The model under review builds one solid part; all positions refer to its coordinate system, in mm. A direction names the side the tool comes from. Round coordinates to 2 decimals unless told otherwise and drop trailing zeros. Loops run counter-clockwise (first coordinate to the right, second up) from the corner with the lowest first, then second, coordinate; pieces in that order, holes last. Notation, with made-up numbers: (31, -23.5) -> (46, -23.5) arc R12 cw to (46, -19.5) -> close; hole circle Ø9 at (56.25, 60.25). An arc over 180 degrees is marked (long way). Use a Markdown table: item, result. Add a question column.
1) Mouldability with a two-part tool opening along Y and no side actions: class faces 1 (the cylindrical face through (31.1, -49, 3.1)), 2 (the flat face through (33.02, -1, 3)), 3 (the cylindrical face through (-31.1, 49, 3.1)), 4 (the cylindrical face through (-18.945, 34.933, 3.131)) as released by +Y, released by -Y, zero draft, split by the parting line, or undercut.
2) Wall thickness on probe 1 along X at (y, z) = (36, 3); probe 2 along Y at (x, z) = (-25, 5); probe 3 along Y at (x, z) = (0, 32): over which ranges is each line inside the solid? List them lowest first.
3) Consider section B-B on x = 0. Give the boundary of the cut face in (y, z).
4) Consider section C-C on y = 23. Give the boundary of the cut face in (x, z), plus the area to 3 significant figures.
5) Consider section D-D on z = 19. Give the boundary of the cut face in (x, y).
6) Insertion check: pin 1 (3 mm diameter, centred on x = -20.5, z = 9, fed in from +Y); pin 2 (1.5 mm diameter, centred on y = -24.5, z = 26, fed in from +X); pin 3 (5 mm diameter, centred on x = 26.5, z = 51, fed in from -Y). Each pin has a flat end and moves straight along its axis. Give the tip position at first contact, or say it passes through.
7) For faces 5 (the flat face through (0, 37, 6.35)), 6 (the cylindrical face through (15.237, -29.294, 33.273)), 7 (the flat face through (0, -36, 6.35)), 8 (the cylindrical face through (2.198, 31.543, 33.875)), list the 3-axis set-ups (+Z, -Z, +X, -X, +Y, -Y) from which the entire face can be reached by the end or side of a thin tool; tool diameter is ignored.
8) Consider section A-A on y = 36.83. Give the boundary of the cut face in (x, z).
from build123d import *

# Parameters (mm, degrees)
F0_R     = 4.953
F0_R_2   = 30.48
F1_DEPTH = 6.35
F2_R     = 33.02
F2_R_2   = 30.48
F3_DEPTH = 54.61
F5_D     = 9.525
F5_DEPTH = 50.801


with BuildPart() as f1:
    # F0 (on Top) → F1 (new body)
    with BuildSketch(Plane.XY):
        with BuildLine():
            ThreePointArc((33.02, 44.45), (31.1601280605, 48.9401280605), (26.67, 50.8))
            Line((26.67, 50.8), (-26.67, 50.8))
            ThreePointArc((-26.67, 50.8), (-31.1601280605, 48.9401280605), (-33.02, 44.45))
            Line((-33.02, 44.45), (-33.02, -44.45))
            ThreePointArc((-33.02, -44.45), (-31.1601280605, -48.9401280605), (-26.67, -50.8))
            Line((-26.67, -50.8), (26.67, -50.8))
            ThreePointArc((26.67, -50.8), (31.1601280605, -48.9401280605), (33.02, -44.45))
            Line((33.02, -44.45), (33.02, 44.45))
        make_face()
        with Locations((-25.4, -36.83)):
            Circle(F0_R, mode=Mode.SUBTRACT)
        with Locations((25.4, -36.83)):
            Circle(F0_R, mode=Mode.SUBTRACT)
        Circle(F0_R_2, mode=Mode.SUBTRACT)
        with Locations((-23.5207291554, 36.83)):
            Circle(F0_R, mode=Mode.SUBTRACT)
        with Locations((25.4, 36.83)):
            Circle(F0_R, mode=Mode.SUBTRACT)
    extrude(amount=F1_DEPTH)

    # F2 (on face) → F3 (join)
    with BuildSketch(Plane.XY.offset(6.35)):
        Circle(F2_R)
        Circle(F2_R_2, mode=Mode.SUBTRACT)
    extrude(amount=F3_DEPTH)

    # F5 (through all, one way)
    with BuildSketch(Plane.XZ):
        with Locations((0, 38.1)):
            Circle(F5_D / 2)
    extrude(amount=-F5_DEPTH, mode=Mode.SUBTRACT)


solid = f1.part
Result set:
| question | item | result |
|---|---|---|
| 1 | face 1 | released by -Y |
| 1 | face 2 | zero draft |
| 1 | face 3 | released by +Y |
| 1 | face 4 | undercut |
| 2 | probe 1 | -33.02 to -28.4, -18.64 to 20.52, 30.28 to 33.02 |
| 2 | probe 2 | -50.8 to -41.77, -31.89 to -17.44, 17.44 to 32.1, 41.56 to 50.8 |
| 2 | probe 3 | -33.02 to -30.48, 30.48 to 33.02 |
| 3 | outline | (-50.8, 0) -> (-30.48, 0) -> (-30.48, 60.96) -> (-33.02, 60.96) -> (-33.02, 6.35) -> (-50.8, 6.35) -> close; (30.48, 0) -> (50.8, 0) -> (50.8, 6.35) -> (33.02, 6.35) -> (33.02, 33.34) -> (30.48, 33.34) -> close; (30.48, 42.86) -> (33.02, 42.86) -> (33.02, 60.96) -> (30.48, 60.96) -> close |
| 4 | outline | (-33.02, 0) -> (-20, 0) -> (-20, 60.96) -> (-23.69, 60.96) -> (-23.69, 6.35) -> (-33.02, 6.35) -> close; (20, 0) -> (33.02, 0) -> (33.02, 6.35) -> (23.69, 6.35) -> (23.69, 60.96) -> (20, 60.96) -> close |
| 4 | area | 569 mm2 |
| 5 | outline | circle Ø66.04 at (0, 0); hole circle Ø60.96 at (0, 0) |
| 6 | pin 1 | y = 27.01 |
| 6 | pin 2 | x = 22.94 |
| 6 | pin 3 | y = -22.68 |
| 7 | face 5 | +Z, +Y |
| 7 | face 6 | +Z |
| 7 | face 7 | +Z, -Y |
| 7 | face 8 | +Y |
| 8 | outline | (-33.02, 0) -> (-28.47, 0) -> (-28.47, 6.35) -> (-33.02, 6.35) -> close; (-18.57, 0) -> (20.45, 0) -> (20.45, 6.35) -> (-18.57, 6.35) -> close; (30.35, 0) -> (33.02, 0) -> (33.02, 6.35) -> (30.35, 6.35) -> close |
